```python
from build123d import *

# Parameters (mm, degrees)
BOSS_EXTRUDE1_DEPTH = 76.2
SKETCH4_R           = 2.54
CUT_EXTRUDE2_DEPTH  = 25.4
SKETCH6_R           = 2.54
CUT_EXTRUDE4_DEPTH  = 25.4


with BuildPart() as part:
    # Sketch1 → Boss-Extrude1 (new body)
    with BuildSketch(Plane(origin=(0, 0, 0), x_dir=(1, 0, 0), z_dir=(0, 1, 0))):
        Polygon((37.11256121, 167.224507406), (-98.77743879, 167.224507406), (-98.77743879, 125.314507406), (-92.42743879, 125.314507406), (-92.42743879, 160.874507406), (30.76256121, 160.874507406), (30.76256121, -4.225492594), (-27.78443879, -4.225492594), (-27.78443879, -10.575492594), (37.11256121, -10.575492594), align=None)
    extrude(amount=BOSS_EXTRUDE1_DEPTH)

    # Sketch4 → Cut-Extrude2 (cut)
    with BuildSketch(Plane.ZY.offset(27.78443879)):
        with Locations((7.400492594, 66.04)):
            Circle(SKETCH4_R)
        with Locations((7.400492594, 53.34)):
            Circle(SKETCH4_R)
        with Locations((7.400492594, 40.64)):
            Circle(SKETCH4_R)
    extrude(amount=-CUT_EXTRUDE2_DEPTH, mode=Mode.SUBTRACT)

    # Sketch6 → Cut-Extrude4 (cut)
    with BuildSketch(Plane.XY.offset(-125.314507406)):
        with Locations((-95.60243879, 66.04)):
            Circle(SKETCH6_R)
        with Locations((-95.60243879, 53.34)):
            Circle(SKETCH6_R)
        with Locations((-95.60243879, 40.64)):
            Circle(SKETCH6_R)
    extrude(amount=-CUT_EXTRUDE4_DEPTH, mode=Mode.SUBTRACT)


solid = part.part
```
Design review of the part built by this model. Coordinates are the model's own, in mm. A direction names the side the tool comes from. Give positions to 0.01 mm unless a question says otherwise; leave off trailing zeros. Write each loop counter-clockwise with the first axis right and the second up, starting at its lowest first coordinate (ties: lowest second). Pieces come first, ordered by that corner, then holes. Notation, with made-up numbers: (42.25, 79) -> (88.25, 79) arc R26 cw to (88.25, 100) -> close; hole circle Ø9 at (45, 45). An arc over 180 degrees is marked (long way). Answer in a Markdown table with one row per item.
(1) For faces 4 (the cylindrical face through (-15.26, 55.06, 5.53)), 5 (the flat face through (-96, 41, -150.715)), 6 (the flat face through (2, 38, 4.225)), 7 (the flat face through (-92.427, 38, -143)), 8 (the flat face through (-32, 38, -160.875)), list the 3-axis set-ups (+Z, -Z, +X, -X, +Y, -Y) from which the entire face can be reached by the end or side of a thin tool; tool diameter is ignored.
Results:
| item | result |
|---|---|
| face 4 | -X |
| face 5 | +Z |
| face 6 | -X, +Y, -Y |
| face 7 | +Z, +Y, -Y |
| face 8 | +Y, -Y |
(2) Mouldability with a two-part tool opening along Z and no side actions: class faces 1 (the flat face through (30.763, 38, -79)), 2 (the flat face through (-96, 66, -150.715)), 3 (the cylindrical face through (-93.18, 41.4, -137.84)) as +Z half, -Z half, draft (parallel to the pull), parting line (faces both ways), or undercut.
Results:
| item | result |
|---|---|
| face 1 | undercut |
| face 2 | +Z half |
| face 3 | draft |
(3) Consider section B-B (z = -140). State the section outline as (x, y) points, then the cut area to 3 significant figures.
Results:
| item | result |
|---|---|
| outline | (-98.78, 0) -> (-92.43, 0) -> (-92.43, 76.2) -> (-98.78, 76.2) -> close; (30.76, 0) -> (37.11, 0) -> (37.11, 76.2) -> (30.76, 76.2) -> close; hole circle Ø5.08 at (-95.6, 40.64); hole circle Ø5.08 at (-95.6, 53.34); hole circle Ø5.08 at (-95.6, 66.04) |
| area | 907 mm2 |
(4) Consider section A-A (x = 23). State the section outline as (y, z) points.
Results:
| item | result |
|---|---|
| outline | (0, -167.22) -> (76.2, -167.22) -> (76.2, -160.87) -> (0, -160.87) -> close; (0, 4.23) -> (76.2, 4.23) -> (76.2, 10.58) -> (0, 10.58) -> close |
(5) Clearance check with flat-ended pins moving along their axes: pin 1 (7 mm diameter, centred on y = 51, z = 8.5, fed in from -X); pin 2 (3 mm diameter, centred on x = -95.6, y = 53.34, fed in from +Z); pin 3 (5.5 mm diameter, centred on x = -97, y = 65, fed in from +Z). State where each tip first meets the part, or that it passes through.
Results:
| item | result |
|---|---|
| pin 1 | x = -27.78 |
| pin 2 | z = -150.71 |
| pin 3 | z = -125.31 |
(6) To check wall thickness, follow probe 1 along Z at (x, y) = (-16, 66); probe 2 along X at (y, z) = (53, -145); probe 3 along Z at (x, y) = (10, 10). State the ranges of each line that lie inside material, in increasing order.
Results:
| item | result |
|---|---|
| probe 1 | -167.22 to -160.87, 4.23 to 4.86, 9.94 to 10.58 |
| probe 2 | -98.78 to -98.12, -93.09 to -92.43, 30.76 to 37.11 |
| probe 3 | -167.22 to -160.87, 4.23 to 10.58 |
(7) Consider section D-D (z = -40). State the section outline as (x, y) points.
Results:
| item | result |
|---|---|
| outline | (30.76, 0) -> (37.11, 0) -> (37.11, 76.2) -> (30.76, 76.2) -> close |
(8) Consider section C-C (y = 40.64). State the section outline as (x, z) points.
Results:
| item | result |
|---|---|
| outline | (-98.78, -167.22) -> (37.11, -167.22) -> (37.11, 10.58) -> (-27.78, 10.58) -> (-27.78, 9.94) -> (-2.38, 9.94) -> (-2.38, 4.86) -> (-27.78, 4.86) -> (-27.78, 4.23) -> (30.76, 4.23) -> (30.76, -160.87) -> (-92.43, -160.87) -> (-92.43, -125.31) -> (-93.06, -125.31) -> (-93.06, -150.71) -> (-98.14, -150.71) -> (-98.14, -125.31) -> (-98.78, -125.31) -> close |
